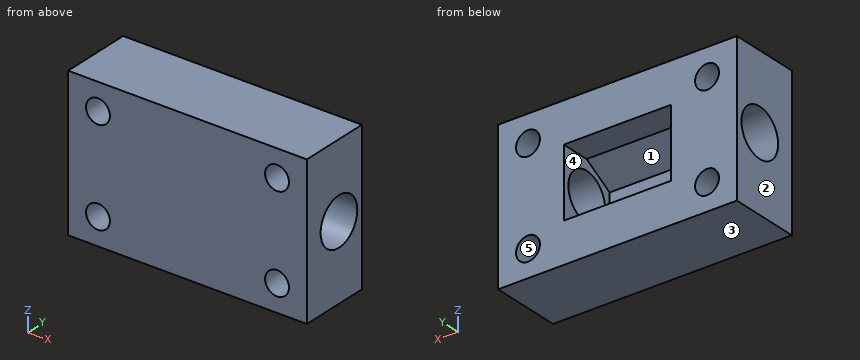
from build123d import *

# Parameters (mm, degrees)
SKETCH1_W               = 40
SKETCH1_H               = 25
BOSS_EXTRUDE1_DEPTH     = 12
CUT_EXTRUDE1_DEPTH      = 9
CUT_EXTRUDE1_DEPTH_BACK = 9
SKETCH3_R               = 4
CUT_EXTRUDE2_DEPTH      = 21
CUT_EXTRUDE2_DEPTH_BACK = 21
SKETCH4_R               = 2
CUT_EXTRUDE3_DEPTH      = 1
CUT_EXTRUDE3_DEPTH_BACK = 13


with BuildPart() as part:
    # Sketch1 → Boss-Extrude1 (new body)
    with BuildSketch(Plane(origin=(0, 0, 0), x_dir=(1, 0, 0), z_dir=(0, 1, 0))):
        Rectangle(SKETCH1_W, SKETCH1_H)
    extrude(amount=BOSS_EXTRUDE1_DEPTH)

    # Sketch2 → Cut-Extrude1 (cut, two sides)
    with BuildSketch(Plane(origin=(0, 0, 0), x_dir=(0, 0, -1), z_dir=(1, 0, 0))) as cut_extrude1_sk:
        Polygon((-2.886751346, 2), (2.886751346, 2), (5.773502692, 7), (5.773502692, 12), (-5.773502692, 12), (-5.773502692, 7), align=None)
    extrude(amount=CUT_EXTRUDE1_DEPTH, mode=Mode.SUBTRACT)
    extrude(cut_extrude1_sk.sketch, amount=-CUT_EXTRUDE1_DEPTH_BACK, mode=Mode.SUBTRACT)

    # Sketch3 → Cut-Extrude2 (cut, two sides)
    with BuildSketch(Plane(origin=(0, 0, 0), x_dir=(0, 0, -1), z_dir=(1, 0, 0))) as cut_extrude2_sk:
        with Locations((0, 7)):
            Circle(SKETCH3_R)
    extrude(amount=CUT_EXTRUDE2_DEPTH, mode=Mode.SUBTRACT)
    extrude(cut_extrude2_sk.sketch, amount=-CUT_EXTRUDE2_DEPTH_BACK, mode=Mode.SUBTRACT)

    # Sketch4 → Cut-Extrude3 (cut, two sides)
    with BuildSketch(Plane(origin=(0, 12, 0), x_dir=(1, 0, 0), z_dir=(0, 1, 0))) as cut_extrude3_sk:
        with Locations((-15, 8)):
            Circle(SKETCH4_R)
        with Locations((15, 8)):
            Circle(SKETCH4_R)
        with Locations((15, -8)):
            Circle(SKETCH4_R)
        with Locations((-15, -8)):
            Circle(SKETCH4_R)
    extrude(amount=CUT_EXTRUDE3_DEPTH, mode=Mode.SUBTRACT)
    extrude(cut_extrude3_sk.sketch, amount=-CUT_EXTRUDE3_DEPTH_BACK, mode=Mode.SUBTRACT)


solid = part.part
The listing builds one solid part. Answer for the finished solid, in the listing's coordinates (mm). Face numbers are marked on the shaded views. A direction names the side the tool comes from. Round coordinates to 2 decimals unless told otherwise and drop trailing zeros. Loops run counter-clockwise (first coordinate to the right, second up) from the corner with the lowest first, then second, coordinate; pieces in that order, holes last. Notation, with made-up numbers: M -22,64.5 L 23,64.5 A28 cw 23,97.5 Z; hole C -8,17.25 d4. An arc over 180 degrees is marked long. Return JSON: item names as keys, results as strings.
Q1. The mould has two halves that part along Z. Classify the marked faces 1, 2 and 3: released by +Z, released by -Z, zero draft, split by the parting line, or undercut.
Results list:
{"face 1": "undercut", "face 2": "zero draft", "face 3": "released by -Z"}
Q2. Find section D-D, the plane x = 11. Determine the outline of the cut face in (y, z), plus the area to 3 significant figures.
Results list:
{"outline": "M 0,-12.5 L 12,-12.5 L 12,12.5 L 0,12.5 Z; hole C 7,0 d8", "area": "250 mm2"}
Q3. Which of the six approach directions +Z, -Z, +X, -X, +Y, -Y give full straight-line access (tool end or side, diameter ignored) to the marked faces 4 and 5?
Results list:
{"face 4": "+Y", "face 5": "+Y, -Y"}
Q4. Each of these flat-tipped pins is pushed along its axis until it touches: pin 1 Ø5 at (x, z) = (15, -8) entering from -Y; pin 2 Ø6.5 at (x, z) = (-0.5, -1) entering from +Y; pin 3 Ø6 at (x, z) = (2, -2.5) entering from +Y. Where does it stop, or does it pass through?
Results list:
{"pin 1": "stops at y = 0", "pin 2": "stops at y = 4.36", "pin 3": "stops at y = 6.53"}
Q5. Find section B-B, the plane z = 0. Determine the outline of the cut face in (x, y).
Results list:
{"outline": "M -20,0 L 20,0 L 20,3 L 9,3 L 9,2 L -9,2 L -9,3 L -20,3 Z; M -20,11 L -9,11 L -9,12 L -20,12 Z; M 9,11 L 20,11 L 20,12 L 9,12 Z"}
Q6. Find the intervals of material crossed by line 1 along Z through (x, y) = (15, 2.75); line 2 along X through (y, z) = (5, -8); line 3 along Z through (x, y) = (15, 7), in increasing order. Write a range as from..to.
Results list:
{"line 1": "z = -12.5..-10, -6..6, 10..12.5", "line 2": "x = -20..-17, -13..13, 17..20", "line 3": "z = -12.5..-10, -6..-4, 4..6, 10..12.5"}
Q7. Find section C-C, the plane y = 11.5. Determine the outline of the cut face in (x, z).
Results list:
{"outline": "M -20,-12.5 L 20,-12.5 L 20,12.5 L -20,12.5 Z; hole C -15,-8 d4; hole C -15,8 d4; hole M -9,-5.77 L 9,-5.77 L 9,5.77 L -9,5.77 Z; hole C 15,-8 d4; hole C 15,8 d4"}
Q8. Find section A-A, the plane x = -15. Determine the outline of the cut face in (y, z), plus the area to 3 significant figures.
Results list:
{"outline": "M 0,-12.5 L 12,-12.5 L 12,-10 L 0,-10 Z; M 0,-6 L 12,-6 L 12,6 L 0,6 Z; M 0,10 L 12,10 L 12,12.5 L 0,12.5 Z; hole C 7,0 d8", "area": "154 mm2"}
